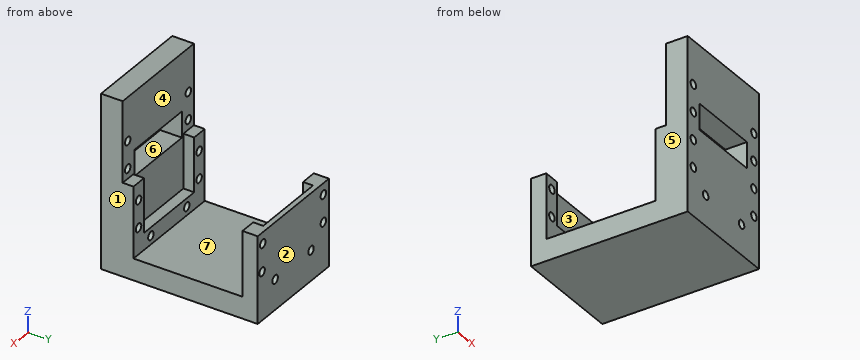
from build123d import *

# Parameters (mm, degrees)
SKETCH1_W                 = 31.75
SKETCH1_H                 = 50.8
BOSS_EXTRUDE1_DEPTH       = 45.974
CUT_EXTRUDE1_DEPTH        = 32.75
SKETCH3_W                 = 22.352
SKETCH3_H                 = 15.875
CUT_EXTRUDE2_DEPTH        = 3.175
SKETCH4_W                 = 31.75
SKETCH4_H                 = 25.4
CUT_EXTRUDE3_DEPTH        = 4.4704
CUT_EXTRUDE4_START        = -1.524
SKETCH5_W                 = 22.225
SKETCH5_H                 = 12.7
CUT_EXTRUDE4_DEPTH        = 2.9464
F_2_CLEARANCE_HOLE1_D     = 2.4384
F_2_CLEARANCE_HOLE1_DEPTH = 9.525
F_2_CLEARANCE_HOLE2_D     = 2.4384
F_2_CLEARANCE_HOLE2_DEPTH = 4.4704
SKETCH10_W                = 21.082
SKETCH10_H                = 7.62
CUT_EXTRUDE5_DEPTH        = 6.35
F_2_CLEARANCE_HOLE3_D     = 2.4384


with BuildPart() as part:
    # Sketch1 → Boss-Extrude1 (new body)
    with BuildSketch(Plane(origin=(0, 0, 0), x_dir=(1, 0, 0), z_dir=(0, 1, 0))):
        Rectangle(SKETCH1_W, SKETCH1_H)
    extrude(amount=BOSS_EXTRUDE1_DEPTH)

    # Sketch2 → Cut-Extrude1 (cut, through all)
    with BuildSketch(Plane.ZY.offset(15.875)):
        Polygon((1.778, 6.35), (25.4, 6.35), (25.4, 41.5036), (-19.05, 41.5036), (-19.05, 9.525), (1.778, 9.525), align=None)
    extrude(amount=-CUT_EXTRUDE1_DEPTH, mode=Mode.SUBTRACT)

    # Sketch3 → Cut-Extrude2 (cut)
    with BuildSketch(Plane(origin=(0, 9.525, 0), x_dir=(1, 0, 0), z_dir=(0, 1, 0))):
        with Locations((0, 6.1595)):
            Rectangle(SKETCH3_W, SKETCH3_H)
    extrude(amount=-CUT_EXTRUDE2_DEPTH, mode=Mode.SUBTRACT)

    # Sketch4 → Cut-Extrude3 (cut)
    with BuildSketch(Plane(origin=(0, 45.974, 0), x_dir=(1, 0, 0), z_dir=(0, 1, 0))):
        with Locations((0, -12.7)):
            Rectangle(SKETCH4_W, SKETCH4_H)
    extrude(amount=-CUT_EXTRUDE3_DEPTH, mode=Mode.SUBTRACT)

    # Sketch5 → Cut-Extrude4 (cut)
    with BuildSketch(Plane(origin=(0, 45.974, 0), x_dir=(1, 0, 0), z_dir=(0, 1, 0)).offset(CUT_EXTRUDE4_START)):
        with Locations((0, 6.35)):
            Rectangle(SKETCH5_W, SKETCH5_H)
    extrude(amount=-CUT_EXTRUDE4_DEPTH, mode=Mode.SUBTRACT)

    # #2 Clearance Hole1
    with Locations(Plane(origin=(0, 9.525, 0), x_dir=(1, 0, 0), z_dir=(0, 1, 0))):
        with Locations((-13.375, 11.3), (-13.375, 3.3), (-7.875, 16.55), (8.125, 16.55), (13.625, 3.3), (13.625, 11.3)):
            Hole(F_2_CLEARANCE_HOLE1_D / 2, depth=F_2_CLEARANCE_HOLE1_DEPTH)

    # #2 Clearance Hole2
    with Locations(Plane(origin=(0, 41.5036, 0), x_dir=(-1, 0, 0), z_dir=(0, -1, 0))):
        with Locations((13.375, 11.3), (7.875, 16.55), (-8.125, 16.55), (-13.932840587, 11.3), (-13.625, 3.3), (13.375, 3.3)):
            Hole(F_2_CLEARANCE_HOLE2_D / 2, depth=F_2_CLEARANCE_HOLE2_DEPTH)

    # Sketch10 → Cut-Extrude5 (cut)
    with BuildSketch(Plane(origin=(0, 6.35, 0), x_dir=(1, 0, 0), z_dir=(0, 1, 0))):
        with Locations((0, -4.767798325)):
            Rectangle(SKETCH10_W, SKETCH10_H)
    extrude(amount=-CUT_EXTRUDE5_DEPTH, mode=Mode.SUBTRACT)

    # #2 Clearance Hole3 (through all)
    with Locations(Plane(origin=(0, 6.35, 0), x_dir=(1, 0, 0), z_dir=(0, 1, 0))):
        with Locations((-13.375, -4.7), (-13.375, -12.7), (13.625, -12.7), (13.625, -4.7)):
            Hole(F_2_CLEARANCE_HOLE3_D / 2)


solid = part.part
Verification items for the finished model (mm, model axes). Face numbers are marked on the shaded views. A direction names the side the tool comes from. Give positions to 0.01 mm unless a question says otherwise; leave off trailing zeros. Write each loop counter-clockwise with the first axis right and the second up, starting at its lowest first coordinate (ties: lowest second). Pieces come first, ordered by that corner, then holes. Notation, with made-up numbers: M 85,22 L 91,22 A32 cw 91,56 Z; hole C 39.25,58.5 d7. An arc over 180 degrees is marked long. Write item = value, one per line.
(1) Access from +Z, -Z, +X, -X, +Y, -Y to the whole of each face (thin tool, end or side, straight path). Record for the marked faces 4, 5, 6 and 7.
Found:
face_4 = +Z
face_5 = +Z, -Z, -X, +Y, -Y
face_6 = +Y, -Y
face_7 = +Z, +X, -X
(2) Material ranges on line 1 (X direction, y = 42, z = -6.5) (1 decimal); line 2 (Z direction, x = -4, y = 4); line 3 (Y direction, x = 2.5, z = -1.5), recorded low to high.
Found:
line_1 = -15.9 to -11.1, 11.1 to 15.9
line_2 = -25.4 to 0.96, 8.58 to 25.4
line_3 = 0 to 6.35, 44.45 to 45.97
(3) Sectioned sample at A-A (z = 4.7). Record the cut outline in (x, y) (3 decimals).
Found:
outline = M -15.875,0 L -14.594,0 L -14.594,6.35 L -15.875,6.35 Z; M -12.156,0 L -10.541,0 L -10.541,6.35 L -12.156,6.35 Z; M 10.541,0 L 12.406,0 L 12.406,6.35 L 10.541,6.35 Z; M 14.844,0 L 15.875,0 L 15.875,6.35 L 14.844,6.35 Z
(4) Sectioned sample at B-B (z = -11.3). Give the number of separate pieces and of enclosed holes in the cut face, then the cut area to 3 significant figures.
Found:
separate_pieces = 6
enclosed_holes = 0
area = 240 mm2
(5) Draft check along Y on the marked faces 1, 2 and 3. Enter one of: released by +Y, released by -Y, zero draft, split by the parting line, or undercut.
Found:
face_1 = zero draft
face_2 = released by +Y
face_3 = undercut
(6) Sectioned sample at D-D (y = 39). Record the cut outline in (x, z) (3 decimals), then the cut area to 3 significant figures.
Found:
outline = M -15.875,-25.4 L 15.875,-25.4 L 15.875,-19.05 L -15.875,-19.05 Z
area = 202 mm2
(7) Sectioned sample at C-C (x = -7.5). Record the cut outline in (y, z) (3 decimals).
Found:
outline = M 0,-25.4 L 45.974,-25.4 L 45.974,-17.71 L 41.504,-17.71 L 41.504,-19.05 L 9.525,-19.05 L 9.525,-17.71 L 0,-17.71 Z; M 0,-15.39 L 9.525,-15.39 L 9.525,-14.097 L 6.35,-14.097 L 6.35,0.958 L 0,0.958 Z; M 0,8.578 L 6.35,8.578 L 6.35,25.4 L 0,25.4 Z; M 41.504,-15.39 L 45.974,-15.39 L 45.974,0 L 44.45,0 L 44.45,-12.7 L 41.504,-12.7 Z
(8) Go/stop test with flat-tipped pins: pin 1 Ø2 at (x, z) = (-7.875, -16.55) entering from -Y; pin 2 Ø8 at (x, y) = (-8, 41) entering from +Z; pin 3 Ø2.5 at (x, y) = (4, 43) entering from +Z; pin 4 Ø1 at (x, y) = (-13.5, 7) entering from +Z. Record where each tip stops, or that it passes through.
Found:
pin_1 = through
pin_2 = 0
pin_3 = -12.7
pin_4 = 1.78
